For this review, take the finished solid that the model builds, in its own axes (mm). Round coordinates to 2 decimals unless told otherwise and drop trailing zeros. Loops run counter-clockwise (first coordinate to the right, second up) from the corner with the lowest first, then second, coordinate; pieces in that order, holes last.
1) Take a section at C-C (z = 3). Give the number of separate pieces and of enclosed holes in the cut face, then the cut area to 3 significant figures.
2) Wall thickness on L1, parallel to Y at x = 0, z = 6; L2, parallel to X at y = 72.5, z = 9.5; L3, parallel to Y at x = -91, z = 2.5: over which ranges is each line inside the solid? List them lowest first.
3) Take a section at A-A (y = 0). State the section outline as (x, z) points, then the cut area to 3 significant figures.
4) Insertion check: pin 1 (2 mm diameter, centred on x = -67.5, z = 2.5, fed in from -Y); pin 2 (7.5 mm diameter, centred on x = -54.68, y = 132, fed in from +Z); pin 3 (1 mm diameter, centred on x = -120, z = 8, fed in from -Y); pin 4 (5 mm diameter, centred on x = -67, z = 6.5, fed in from -Y). Each pin has a flat end and moves straight along its axis. Give the tip position at first contact, or say it passes through.
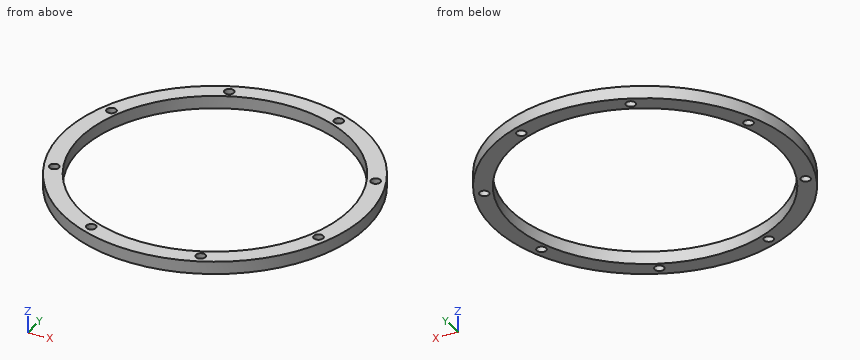
```python
from build123d import *

# Parameters (mm, degrees)
F0_R     = 152.4
F0_R_2   = 4.7625
F0_R_3   = 134.9375
F1_DEPTH = 12.7


with BuildPart() as f1:
    # F0 (on Top) → F1 (new body)
    with BuildSketch(Plane.XY):
        Circle(F0_R)
        with Locations((-54.675895, -131.999288)):
            Circle(F0_R_2, mode=Mode.SUBTRACT)
        with Locations((-131.999288, -54.675895)):
            Circle(F0_R_2, mode=Mode.SUBTRACT)
        with Locations((54.675895, -131.999288)):
            Circle(F0_R_2, mode=Mode.SUBTRACT)
        with Locations((131.999288, -54.675895)):
            Circle(F0_R_2, mode=Mode.SUBTRACT)
        with Locations((-131.999288, 54.675895)):
            Circle(F0_R_2, mode=Mode.SUBTRACT)
        with Locations((-54.675895, 131.999288)):
            Circle(F0_R_2, mode=Mode.SUBTRACT)
        Circle(F0_R_3, mode=Mode.SUBTRACT)
        with Locations((131.999288, 54.675895)):
            Circle(F0_R_2, mode=Mode.SUBTRACT)
        with Locations((54.675895, 131.999288)):
            Circle(F0_R_2, mode=Mode.SUBTRACT)
    extrude(amount=F1_DEPTH)


solid = f1.part
```
Response:
1. separate pieces: 1
1. enclosed holes: 9
1. area: 15,200 mm2
2. L1: y = -152.4 to -134.94, 134.94 to 152.4
2. L2: x = -134.05 to -113.81, 113.81 to 134.05
2. L3: y = -122.25 to -99.63, 99.63 to 122.25
3. outline: (-152.4, 0) - (-134.94, 0) - (-134.94, 12.7) - (-152.4, 12.7) - close; (134.94, 0) - (152.4, 0) - (152.4, 12.7) - (134.94, 12.7) - close
3. area: 444 mm2
4. pin 1: stops at y = -137.13
4. pin 2: passes through
4. pin 3: stops at y = -94.58
4. pin 4: stops at y = -138.08
